Can you work these out from the model? Positions are in its coordinate system, mm. A direction names the side the tool comes from. Coordinates: 2 decimals unless noted, no trailing zeros. Write each loop counter-clockwise with the first axis right and the second up, starting at its lowest first coordinate (ties: lowest second). Pieces come first, ordered by that corner, then holes. Notation, with made-up numbers: M -28.5,86 L -8.5,86 A27 ccw -8.5,106 Z; hole C -40,21.25 d1. An arc over 180 degrees is marked long. Answer as a JSON object with one key per item and string values. Group by question number.
from build123d import *

# Parameters (mm, degrees)
F0_R      = 19.5
F1_DEPTH  = 7.5
F3_R      = 17.5
F4_DEPTH  = 2
F2_R      = 17.5
F5_DEPTH  = 2
F6_R      = 1.5
F7_DEPTH  = 25
F8_R      = 17.5
F8_R_2    = 2.5
F9_DEPTH  = 4
F10_R     = 17.5
F10_R_2   = 2.5
F11_DEPTH = 4


with BuildPart() as f1:
    # F0 (on Right) → F1 (new body, symmetric)
    with BuildSketch(Plane.YZ):
        Circle(F0_R)
    extrude(amount=F1_DEPTH, both=True)

    # F3 (on face) → F4 (cut)
    with BuildSketch(Plane(origin=(-7.5, 0, 0), x_dir=(0, -1, 0), z_dir=(-1, 0, 0))):
        Circle(F3_R)
    extrude(amount=-F4_DEPTH, mode=Mode.SUBTRACT)

    # F2 (on face) → F5 (cut)
    with BuildSketch(Plane.YZ.offset(7.5)):
        Circle(F2_R)
    extrude(amount=-F5_DEPTH, mode=Mode.SUBTRACT)

    # F6 (on face) → F7 (cut)
    with BuildSketch(Plane.YZ.offset(5.5)):
        Circle(F6_R)
    extrude(amount=-F7_DEPTH, mode=Mode.SUBTRACT)

    # F8 (on face) → F9 (cut)
    with BuildSketch(Plane.YZ.offset(5.5)):
        Circle(F8_R)
        Circle(F8_R_2, mode=Mode.SUBTRACT)
    extrude(amount=-F9_DEPTH, mode=Mode.SUBTRACT)

    # F10 (on face) → F11 (cut)
    with BuildSketch(Plane(origin=(-5.5, 0, 0), x_dir=(0, -1, 0), z_dir=(-1, 0, 0))):
        Circle(F10_R)
        Circle(F10_R_2, mode=Mode.SUBTRACT)
    extrude(amount=-F11_DEPTH, mode=Mode.SUBTRACT)


solid = f1.part
Q1. Will these pins go through, and if not, where does the flat tip stop? pin 1 (4 mm diameter, centred on x = -5.5, z = -15.5, fed in from +Y); pin 2 (21 mm diameter, centred on y = 0, z = 0, fed in from -X); pin 3 (4 mm diameter, centred on x = -5, y = -6, fed in from -Z).
Q2. If we section it at C-C on x = -2.25: List the corners of the cut face in (y, z) for me.
Q3. If we section it at D-D on y = 7.5: List the corners of the cut face in (x, z) for me, and give its area (3 significant figures).
Q4. We'd pull the mould along Z, two halves only. Please class faces 4 (the cylindrical face through (0.105, -2.539, 19.334)), 5 (the cylindrical face through (0.08, -1.5, 0.07)), 6 (the flat face through (7.5, -13, 12)): pulls with the +Z half, pulls with the -Z half, needs draft (parallel to the pull), parting line crosses it, or undercut.
Q5. On a 3-axis mill with a long thin cutter (end or side, diameter ignored), from which of +Z, -Z, +X, -X, +Y, -Y can I reach the whole of each face in a straight line? I mean faces 1 (the flat face through (-1.5, 0, -4)), 2 (the cylindrical face through (3.53, -0.54, -2.44)), 3 (the flat face through (-7.5, -13, 12)). Say none if no direction works.
Q6. Please list where these lines run through material, in increasing order: L1, parallel to Z at x = -4.95, y = 0; L2, parallel to Y at x = 5, z = 0.5; L3, parallel to Y at x = 3.25, z = 6.
Q7. If we section it at A-A on z = 0: List the corners of the cut face in (x, y) for me.
Reply:
{
 "1": {"pin 1": "y = 14.07", "pin 2": "x = -5.5", "pin 3": "z = -19.09"},
 "2": {"outline": "C 0,0 d39; C 0,0 d5; hole C 0,0 d35; hole C 0,0 d3"},
 "3": {"outline": "M -7.5,-18 L 7.5,-18 L 7.5,-15.81 L 1.5,-15.81 L 1.5,15.81 L 7.5,15.81 L 7.5,18 L -7.5,18 L -7.5,15.81 L -1.5,15.81 L -1.5,-15.81 L -7.5,-15.81 Z", "area": "161 mm^2"},
 "4": {"face 4": "parting line crosses it", "face 5": "undercut", "face 6": "needs draft"},
 "5": {"face 1": "-X", "face 2": "+X", "face 3": "+Z, -Z, -X, +Y, -Y"},
 "6": {"L1": "-19.5 to -17.5, -2.5 to -1.5, 1.5 to 2.5, 17.5 to 19.5", "L2": "-19.49 to -17.49, -2.45 to -1.41, 1.41 to 2.45, 17.49 to 19.49", "L3": "-18.55 to -16.44, 16.44 to 18.55"},
 "7": {"outline": "M -7.5,-19.5 L 7.5,-19.5 L 7.5,-17.5 L 1.5,-17.5 L 1.5,-2.5 L 5.5,-2.5 L 5.5,-1.5 L -5.5,-1.5 L -5.5,-2.5 L -1.5,-2.5 L -1.5,-17.5 L -7.5,-17.5 Z; M -7.5,17.5 L -1.5,17.5 L -1.5,2.5 L -5.5,2.5 L -5.5,1.5 L 5.5,1.5 L 5.5,2.5 L 1.5,2.5 L 1.5,17.5 L 7.5,17.5 L 7.5,19.5 L -7.5,19.5 Z"}
}
